Check sheet for the modelled part. Datum: model origin and axes. Units: mm. Face numbers are marked on the shaded views. Round coordinates to 2 decimals unless told otherwise and drop trailing zeros. Write each loop counter-clockwise with the first axis right and the second up, starting at its lowest first coordinate (ties: lowest second). Pieces come first, ordered by that corner, then holes. Notation, with made-up numbers: M 47,9.25 L 89,9.25 A22 cw 89,36.25 Z; hole C 42,27.25 d5. An arc over 180 degrees is marked long. Answer in a Markdown table with one row per item.
```python
from build123d import *

# Parameters (mm, degrees)
F0_R     = 18.707853832
F1_DEPTH = 127
F3_D     = 25.4


# Not quite as in the source:
# - a fillet or chamfer that OpenCascade refuses, or shapes differently, is made with other operations: its cross-section is extruded or revolved along the edge and cut away or added


with BuildPart() as f1:
    # F0 (on Front) → F1 (new body)
    with BuildSketch(Plane.XZ):
        Circle(F0_R)
    extrude(amount=-F1_DEPTH)

    # F3 (through all)
    with Locations(Plane.XZ):
        with Locations((0, 0)):
            Hole(F3_D / 2)

    # F4: fillet of radius 12.7 on 1 edges, made by hand

    # F4_s1 → F4_t2 (revolve, cut)
    with BuildSketch(Plane.XY):
        with BuildLine():
            ThreePointArc((18.707853832, 10.7937565132), (17.1047060058, 4.6171982618), (12.7, 0))
            Line((12.7, 0), (18.707853832, 0))
            Line((18.707853832, 0), (18.707853832, 10.7937565132))
        make_face()
    revolve(axis=Axis((0, 0, 0), (0, -1, 0)), mode=Mode.SUBTRACT)


solid = f1.part
```
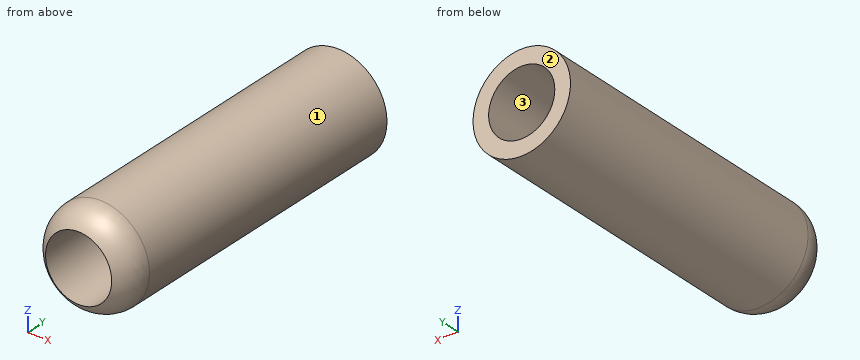
1. Section check A-A, the plane y = 51. Record the cut outline in (x, z), and give its area (3 significant figures).
Found:
| item | result |
|---|---|
| outline | C 0,0 d37.42; hole C 0,0 d25.4 |
| area | 593 mm2 |
2. Go/stop test with flat-tipped pins: pin 1 (2 mm diameter, centred on x = 0, y = 17, fed in from -Z); pin 2 (2 mm diameter, centred on x = -11.5, y = 73.5, fed in from +Z); pin 3 (5 mm diameter, centred on y = 23.5, z = -6.5, fed in from +X). Record where each tip stops, or that it passes through.
Found:
| item | result |
|---|---|
| pin 1 | stops at z = -18.71 |
| pin 2 | stops at z = 15.48 |
| pin 3 | stops at x = 18.28 |
3. Scan lines: L1, parallel to Z at x = 0, y = 73.5; L2, parallel to Y at x = 9, z = -9; L3, parallel to X at y = 68, z = 5. Record each from-to range of solid material in increasing order.
Found:
| item | result |
|---|---|
| L1 | z = -18.71 to -12.7, 12.7 to 18.71 |
| L2 | y = 0.02 to 127 |
| L3 | x = -18.03 to -11.67, 11.67 to 18.03 |
4. Draft check along X on the marked faces 1, 2 and 3. Enter one of: +X half, -X half, draft (parallel to the pull), parting line (faces both ways), or undercut.
Found:
| item | result |
|---|---|
| face 1 | parting line |
| face 2 | draft |
| face 3 | undercut |
